Could you check a few things on this model? Use its own coordinates, in mm. A direction names the side the tool comes from. Give positions to 0.01 mm unless a question says otherwise; leave off trailing zeros. Loops run counter-clockwise (first coordinate to the right, second up) from the corner with the lowest first, then second, coordinate; pieces in that order, holes last. Notation, with made-up numbers: M 25.5,-32 L 72.5,-32 A8 ccw 72.5,-28 Z; hole C 77.25,51.25 d8. An arc over 180 degrees is marked long. Return JSON: item names as keys, results as strings. Group by question number.
1. If we section it at C-C (x = 40): Write out the boundary of the cut face in (y, z).
2. If we section it at B-B (y = -20): Write out the boundary of the cut face in (x, z), plus the area to 3 significant figures.
3. If we mould it in two halves opening along X, with no side actions, what happens to faces 5 (the cylindrical face through (40, -21, 38)), 6 (the flat face through (0, 2, 37)), 7 (the cylindrical face through (41.754, -20.962, 37.542)), 8 (the flat face through (36, -11, 34.5))? For each: +X half, -X half, draft (parallel to the pull), parting line (faces both ways), or undercut.
4. If we section it at D-D (y = -13): Write out the boundary of the cut face in (x, z), plus the area to 3 significant figures.
5. Please list where these lines run through material, in increasing order: line 1 (Y direction, x = 40, z = 37.2); line 2 (Y direction, x = 3.5, z = 68); line 3 (Z direction, x = 37, y = -13).
6. If we section it at A-A (z = 37.5): Write out the boundary of the cut face in (x, y), plus the area to 3 significant figures.
7. For pin 1 (4.5 mm diameter, centred on x = 38.5, y = -6.5, fed in from -Z); pin 2 (7 mm diameter, centred on x = 36.5, y = -13, fed in from +Z); pin 3 (8 mm diameter, centred on x = 37, y = 2, fed in from -Z), each with a flat end and sliding along its axis, tell me the tip position at first contact or that it passes through.
8. For faces 1 (the flat face through (33.38, -9, 38)), 2 (the flat face through (36, -11, 40.5)), 3 (the flat face through (37.38, -8, 38)), 4 (the flat face through (14, 5, 37)), which set-ups out of +Z, -Z, +X, -X, +Y, -Y let a thin tool reach every point of the face, with its end or its side?
```python
from build123d import *

# Parameters (mm, degrees)
AUFSATZ_LINEAR_AUSTRAGEN1_DEPTH = 5
AUFSATZ_LINEAR_AUSTRAGEN2_DEPTH = 6
SKIZZE13_R                      = 1
SCHNITT_LINEAR_AUSTRAGEN1_DEPTH = 6


with BuildPart() as part:
    # Skizze1 → Aufsatz-Linear austragen1 (new body)
    with BuildSketch(Plane(origin=(0, 0, 0), x_dir=(1, 0, 0), z_dir=(0, 1, 0))):
        with BuildLine():
            Line((0, 0), (0, -75))
            ThreePointArc((0, -75), (37.5, -37.5), (0, 0))
        make_face()
    extrude(amount=AUFSATZ_LINEAR_AUSTRAGEN1_DEPTH)

    # Skizze12 → Aufsatz-Linear austragen2 (add)
    with BuildSketch(Plane(origin=(37.379807383, 0, 40.5), x_dir=(1, 0, 0), z_dir=(0, 0, 1))):
        with BuildLine():
            Line((0, 0), (0, -16.177830011))
            Line((0, -16.177830011), (3.620192617, -18.267949192))
            ThreePointArc((3.620192617, -18.267949192), (4.352243424, -21), (1.620192617, -21.732050808))
            Line((1.620192617, -21.732050808), (-4, -18.487231087))
            Line((-4, -18.487231087), (-4, 0))
            Line((-4, 0), (0, 0))
        make_face()
    extrude(amount=-AUFSATZ_LINEAR_AUSTRAGEN2_DEPTH)

    # Skizze13 → Schnitt-Linear austragen1 (cut)
    with BuildSketch(Plane(origin=(37.379807383, 0, 40.5), x_dir=(1, 0, 0), z_dir=(0, 0, 1))):
        with Locations((2.620192617, -20)):
            Circle(SKIZZE13_R)
    extrude(amount=-SCHNITT_LINEAR_AUSTRAGEN1_DEPTH, mode=Mode.SUBTRACT)


solid = part.part
```
Answer:
{
 "1": {"outline": "M -22,34.5 L -21,34.5 L -21,40.5 L -22,40.5 Z; M -19,34.5 L -17.69,34.5 L -17.69,40.5 L -19,40.5 Z"},
 "2": {"outline": "M 36,34.5 L 39,34.5 L 39,40.5 L 36,40.5 Z; M 41,34.5 L 42,34.5 L 42,40.5 L 41,40.5 Z", "area": "24.0 mm²"},
 "3": {"face 5": "undercut", "face 6": "-X half", "face 7": "parting line", "face 8": "draft"},
 "4": {"outline": "M 33.38,34.5 L 37.38,34.5 L 37.38,40.5 L 33.38,40.5 Z", "area": "24.0 mm²"},
 "5": {"line 1": "y = -22 to -21, -19 to -17.69", "line 2": "y = 0 to 5", "line 3": "z = 34.5 to 40.5"},
 "6": {"outline": "M 0,0 L 33.38,0 L 33.38,-18.49 L 39,-21.73 A2 ccw 41,-18.27 L 37.38,-16.18 L 37.38,0 L 37.5,0 L 37.5,5 L 0,5 Z; hole C 40,-20 d2", "area": "281 mm²"},
 "7": {"pin 1": "stops at z = 34.5", "pin 2": "stops at z = 40.5", "pin 3": "stops at z = 19.69"},
 "8": {"face 1": "+Z, -Z, -X, -Y", "face 2": "+Z, +X, -X, -Y", "face 3": "+Z, -Z, +X", "face 4": "+Z, -Z, +X, -X, +Y"}
}
